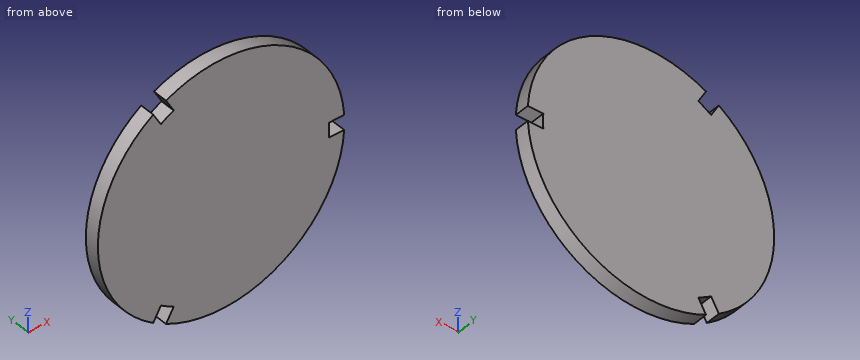
from build123d import *

# Parameters (mm, degrees)
SKETCH1_W           = 88.9
SKETCH1_H           = 12.192
BOSS_EXTRUDE1_DEPTH = 12.192


with BuildPart() as part:
    # Sketch1 → Revolve1 (revolve)
    with BuildSketch(Plane.XY, mode=Mode.PRIVATE) as revolve1_sk:
        with Locations((44.45, -142.376222222)):
            Rectangle(SKETCH1_W, SKETCH1_H)
    revolve(revolve1_sk.sketch.rotate(Axis((0, 0, 0), (0, -1, 0)), 180), axis=Axis((0, 0, 0), (0, -1, 0)))

    # Sketch2 → Boss-Extrude1 (add)
    with BuildSketch(Plane(origin=(0, -136.280222222, 0), x_dir=(1, 0, 0), z_dir=(0, 1, 0))):
        with BuildLine():
            Line((101.416955111, 6.096), (88.716955111, 6.096))
            Line((88.716955111, 6.096), (88.716955111, -6.096))
            Line((88.716955111, -6.096), (101.416955111, -6.096))
            ThreePointArc((101.416955111, -6.096), (50.8, -87.988181024), (-45.429186694, -90.877659501))
            Line((-45.429186694, -90.877659501), (-39.079186694, -79.879136873))
            Line((-39.079186694, -79.879136873), (-49.637768417, -73.783136873))
            Line((-49.637768417, -73.783136873), (-55.987768417, -84.781659501))
            ThreePointArc((-55.987768417, -84.781659501), (-101.6, 0), (-55.987768417, 84.781659501))
            Line((-55.987768417, 84.781659501), (-49.637768417, 73.783136873))
            Line((-49.637768417, 73.783136873), (-39.079186694, 79.879136873))
            Line((-39.079186694, 79.879136873), (-45.429186694, 90.877659501))
            ThreePointArc((-45.429186694, 90.877659501), (50.8, 87.988181024), (101.416955111, 6.096))
        make_face()
    extrude(amount=-BOSS_EXTRUDE1_DEPTH)


solid = part.part
For this review, take the finished solid that the model builds, in its own axes (mm). Round coordinates to 2 decimals unless told otherwise and drop trailing zeros. Loops run counter-clockwise (first coordinate to the right, second up) from the corner with the lowest first, then second, coordinate; pieces in that order, holes last. Notation, with made-up numbers: (82.25, 36) - (94.25, 36) arc R17 ccw to (94.25, 57) - close; hole circle Ø5 at (-14, 42.25). An arc over 180 degrees is marked (long way). Put each result on its own line as item: value. Start each with the question number.
1. Consider section A-A on y = -140.5. State the section outline as (x, z) points, plus the area to 3 significant figures.
2. Insertion check: P1, Ø5, axis at y = -146, z = 71.5, coming from the +X side; P2, Ø6, axis at x = 96, y = -141.5, coming from the -Z side; P3, Ø3.5, axis at x = 94, y = -144, coming from the +Z side. Each pin has a flat end and moves straight along its axis. Give the tip position at first contact, or say it passes through.
3. Consider section B-B on x = 52. State the section outline as (y, z) points.
4. For probe 1 along X at (y, z) = (-145.5, 45.5); probe 2 along Z at (x, y) = (-43.5, -142.25); probe 3 along X at (y, z) = (-138, -80.5), list the stretches that pass through material, from the lowest coordinate up. Write a range as [from, to].
5. Consider section C-C on z = 37.5. State the section outline as (x, y) points.
Result sheet:
1. outline: (-55.99, -84.78) - (-49.64, -73.78) - (-49.3, -73.98) arc R88.9 ccw to (-39.42, -79.68) - (-39.08, -79.88) - (-45.43, -90.88) arc R101.6 ccw to (101.42, -6.1) - (88.72, -6.1) - (88.72, -5.7) arc R88.9 ccw to (88.72, 5.7) - (88.72, 6.1) - (101.42, 6.1) arc R101.6 ccw to (-45.43, 90.88) - (-39.08, 79.88) - (-39.42, 79.68) arc R88.9 ccw to (-49.3, 73.98) - (-49.64, 73.78) - (-55.99, 84.78) arc R101.6 ccw to start
1. area: 32,000 mm^2
2. P1: x = 74.58
2. P2: z = -40.91
2. P3: z = 42.57
3. outline: (-148.47, -87.28) - (-136.28, -87.28) - (-136.28, 87.28) - (-148.47, 87.28) - close
4. probe 1: [-90.84, 90.84]
4. probe 2: [-91.82, -87.54], [-77.53, 77.53], [87.54, 91.82]
4. probe 3: [-61.99, -53.52], [-39.44, 61.99]
5. outline: (-94.43, -148.47) - (94.43, -148.47) - (94.43, -136.28) - (-94.43, -136.28) - close
